```python
from build123d import *

# Parameters (mm, degrees)
F1_DEPTH = 12.7
F2_DEPTH = 12.7
F3_SIZE2 = 12.7
F3_SIZE  = 35.92068


with BuildPart() as f1:
    # F0 (on Top) → F1 (new body)
    with BuildSketch(Plane.XY):
        Polygon((-254.6055446911, 67.5657510931), (-196.2338046911, 9.1940110931), (-45.1038046911, 9.1940110931), (13.2679353089, 67.5657510931), align=None)
    extrude(amount=F1_DEPTH)

    # F0 (on Top) → F2 (join)
    with BuildSketch(Plane.XY):
        Polygon((-254.6055446911, 67.5657510931), (-196.2338046911, 9.1940110931), (-45.1038046911, 9.1940110931), (13.2679353089, 67.5657510931), align=None)
        Polygon((-297.8338046911, 110.7940110931), (-254.6055446911, 67.5657510931), (13.2679353089, 67.5657510931), (56.4961953089, 110.7940110931), align=None)
    extrude(amount=-F2_DEPTH)

    # F3
    f3_edges = [f1.edges().sort_by_distance(p)[0] for p in [
        (-120.668805, 9.194011, 12.7),
    ]]
    f3_side = f1.faces().sort_by_distance((-120.668805, 41.090487, 12.7))[0]
    chamfer(f3_edges, length=F3_SIZE, length2=F3_SIZE2, reference=f3_side)


solid = f1.part
```
Model file for the job. Use its own axes, mm. A direction names the side the tool comes from. Give positions to 0.01 mm unless a question says otherwise; leave off trailing zeros. Write each loop counter-clockwise with the first axis right and the second up, starting at its lowest first coordinate (ties: lowest second). Pieces come first, ordered by that corner, then holes. Notation, with made-up numbers: (0, 29) - (48, 29) arc R29 ccw to (48, 62) - close; hole circle Ø3 at (-2, 20). An arc over 180 degrees is marked (long way). One line per question, with ' | ' between items. Start each with the question number.
(1) Pin check, flat tips, straight feed: P1, Ø1.5, axis at y = 45.5, z = 10, coming from the -X side; P2, Ø3, axis at x = -210, y = 40, coming from the +Z side; P3, Ø6.5, axis at x = -143.5, z = 3.5, coming from the +Y side. Stop position of each tip, or through.
(2) Slice it at A-A on x = -174. Write the cut outline in (y, z), plus the area to 3 significant figures.
(3) Slice it at D-D on x = -13. Write the cut outline in (y, z), plus the area to 3 significant figures.
(4) Wall check: line 1 along Z through (x, y) = (-181.5, 15); line 2 along Z through (x, y) = (-197.5, 102); line 3 along X through (y, z) = (82, -5.75). Give the ranges that are in metal, low to high. Write a range as from..to.
(5) 3-axis set-ups, long thin cutter, end or side, ignore diameter. For faces 1 (the face through (5, 59.3, -2.6)), 2 (the face through (-119, 67.566, 6)): which of +Z, -Z, +X, -X, +Y, -Y reach the whole face in a straight line?
(6) Slice it at B-B on z = -5.75. Write the cut outline in (x, y).
(7) Slice it at C-C on y = 96.5. Write the cut outline in (x, z).
Results below:
1) P1: x = -233.29 | P2: z = 11.42 | P3: y = 67.57
2) outline: (9.19, -12.7) - (110.79, -12.7) - (110.79, 0) - (67.57, 0) - (67.57, 12.7) - (45.11, 12.7) - (9.19, 0) - close | area: 1,800 mm^2
3) outline: (41.3, -12.7) - (110.79, -12.7) - (110.79, 0) - (67.57, 0) - (67.57, 12.7) - (45.11, 12.7) - (41.3, 11.35) - close | area: 1,210 mm^2
4) line 1: -12.7..2.05 | line 2: -12.7..0 | line 3: -269.04..27.7
5) face 1: +Z, -Z, +X, -Y | face 2: +Z, +X, -X, +Y
6) outline: (-297.83, 110.79) - (-196.23, 9.19) - (-45.1, 9.19) - (56.5, 110.79) - close
7) outline: (-283.54, -12.7) - (42.2, -12.7) - (42.2, 0) - (-283.54, 0) - close
